Geometry: see drawing. Coordinates: mm, zero at the bounding-box minimum. A direction names the side the tool comes from. Coordinates: 2 decimals unless noted, no trailing zeros. Loops run counter-clockwise (first coordinate to the right, second up) from the corner with the lowest first, then second, coordinate; pieces in that order, holes last.
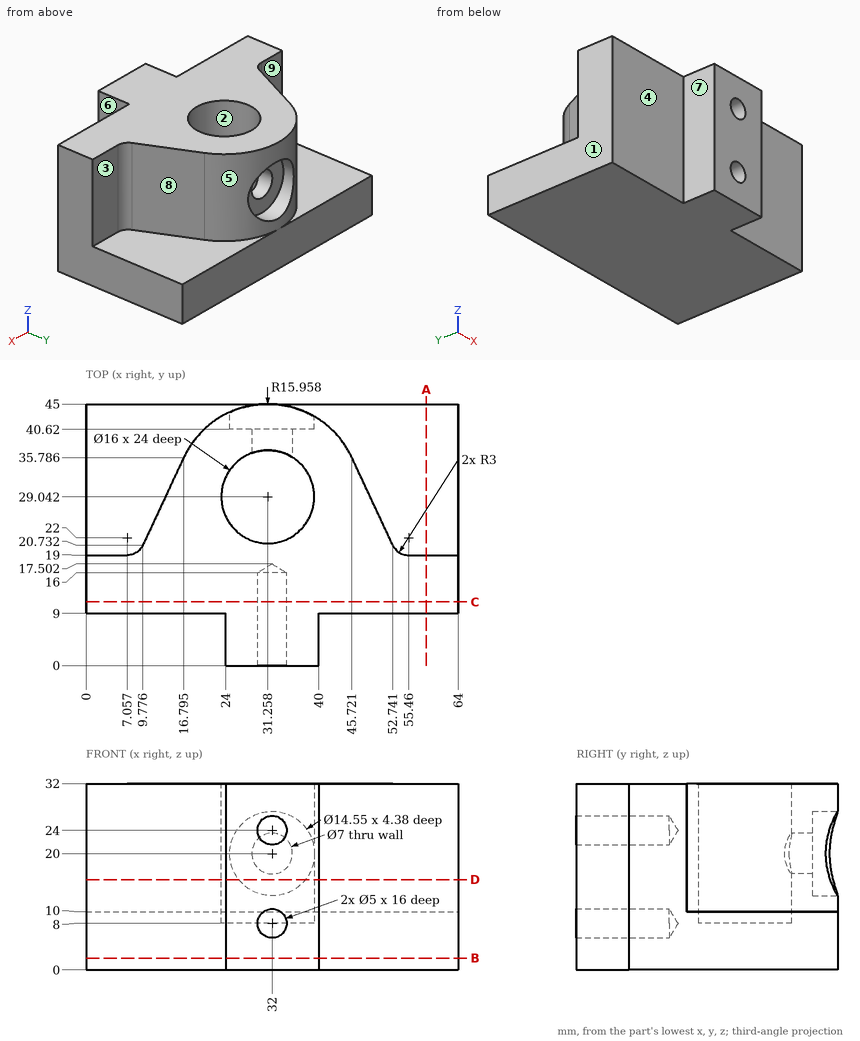
Item 1: Mould query, pull axis Y, two halves, no side actions, for the marked faces 1, 2, 3 and 4. Classes: +Y half, -Y half, draft (parallel to the pull), parting line (faces both ways), or undercut.
Result:
face 1: draft
face 2: undercut
face 3: +Y half
face 4: -Y half
Item 2: Section query C-C (y = 11). Output: boundary loops of the cut face in (x, z), then the cut area to 3 significant figures.
Result:
outline: (0, 0) - (64, 0) - (64, 32) - (0, 32) - close; hole circle Ø5 at (32, 8); hole circle Ø5 at (32, 24)
area: 2,010 mm2
Item 3: Section query D-D (z = 15.5). Output: boundary loops of the cut face in (x, y) (1 decimal), then the cut area to 3 significant figures.
Result:
outline: (0, 9) - (24, 9) - (24, 0) - (40, 0) - (40, 9) - (64, 9) - (64, 19) - (55.5, 19) arc R3 cw to (52.7, 20.7) - (45.7, 35.8) arc R16 ccw to (37.7, 43.6) - (37.7, 40.6) - (26.3, 40.6) - (26.3, 44.2) arc R16 ccw to (16.8, 35.8) - (9.8, 20.7) arc R3 cw to (7.1, 19) - (0, 19) - close; hole circle Ø16 at (31.3, 29)
area: 1,350 mm2
Item 4: Section query B-B (z = 2). Output: boundary loops of the cut face in (x, y), then the cut area to 3 significant figures.
Result:
outline: (0, 9) - (24, 9) - (24, 0) - (40, 0) - (40, 9) - (64, 9) - (64, 45) - (0, 45) - close
area: 2,450 mm2
Item 5: Contact query for flat-ended pins moving along their axis: P1, Ø7, axis at x = 51, z = 14.5, coming from the -Y side; P2, Ø14.5, axis at x = 31.26, y = 29.04, coming from the +Z side; P3, Ø1, axis at x = 23, z = 26.5, coming from the +Y side. Output: stop coordinate, or through.
Result:
P1: stops at y = 9
P2: stops at z = 8
P3: stops at y = 42.99
Item 6: Line query: L1, parallel to Z at x = 32, y = 8.5; L2, parallel to Z at x = 32, y = 43.75 (1 decimal); L3, parallel to Y at x = 22, z = 8. Output: solid intervals per line, ascending.
Result:
L1: z = 0 to 5.5, 10.5 to 21.5, 26.5 to 32
L2: z = 0 to 12.7, 27.3 to 32
L3: y = 9 to 45
Item 7: Reachability of the marked faces 5, 6, 7, 8 and 9 from +Z, -Z, +X, -X, +Y, -Y: full face, straight path, thin tool, end or side. Return the list, or none.
Result:
face 5: +Z, +Y
face 6: +Z, -Z, +X, -Y
face 7: +Z, -Z, -X, -Y
face 8: +Z, +X, +Y
face 9: +Z, -X, +Y
Item 8: Section query A-A (x = 58.5). Output: boundary loops of the cut face in (y, z), then the cut area to 3 significant figures.
Result:
outline: (9, 0) - (45, 0) - (45, 10) - (19, 10) - (19, 32) - (9, 32) - close
area: 580 mm2
